Read the model definition and answer for the solid it produces. Units are mm, in the model's axes. Give positions to 0.01 mm unless a question says otherwise; leave off trailing zeros. Loops run counter-clockwise (first coordinate to the right, second up) from the corner with the lowest first, then second, coordinate; pieces in that order, holes last. Notation, with made-up numbers: (22.25, -16.75) - (59.25, -16.75) arc R24 cw to (59.25, 5.25) - close; hole circle Ø3 at (87, 61). An arc over 180 degrees is marked (long way). Write item = value, one per line.
```python
from build123d import *

# Parameters (mm, degrees)
BOSS_EXTRU_1_DEPTH = 19
CHANFREIN1_SIZE    = 1.5


with BuildPart() as part:
    # Esquisse1 → Boss.-Extru.1 (new body)
    with BuildSketch(Plane.XY):
        Polygon((-4, 0), (4, 0), (4, -2), (2.5, -3.5), (-2.5, -3.5), (-4, -2), align=None)
    extrude(amount=BOSS_EXTRU_1_DEPTH)

    # Chanfrein1
    chanfrein1_edges = [part.edges().sort_by_distance(p)[0] for p in [
        (0, -3.5, 0),
        (0, -3.5, 19),
    ]]
    chamfer(chanfrein1_edges, length=CHANFREIN1_SIZE)


solid = part.part
```
1) A cutting plane is placed at A-A on z = 12.5. Determine the outline of the cut face in (x, y), then the cut area to 4 significant figures.
Output:
outline = (-4, -2) - (-2.5, -3.5) - (2.5, -3.5) - (4, -2) - (4, 0) - (-4, 0) - close
area = 25.75 mm²
2) A cutting plane is placed at B-B on y = -2.6. Determine the outline of the cut face in (x, z), then the cut area to 3 significant figures.
Output:
outline = (-3.4, 0.6) - (3.4, 0.6) - (3.4, 18.4) - (-3.4, 18.4) - close
area = 121 mm²
3) A cutting plane is placed at C-C on x = -1.5. Determine the outline of the cut face in (y, z).
Output:
outline = (-3.5, 1.5) - (-2, 0) - (0, 0) - (0, 19) - (-2, 19) - (-3.5, 17.5) - close
4) Find the intervals of material crossed by probe 1 along Y at (x, z) = (3.5, 18.25); probe 2 along Z at (x, y) = (-1.5, -2.85); probe 3 along Z at (x, y) = (2, -2.3), in increasing order.
Output:
probe_1 = -2.5 to 0
probe_2 = 0.85 to 18.15
probe_3 = 0.3 to 18.7
